Can you work these out from the model? Positions are in its coordinate system, mm. A direction names the side the tool comes from. Coordinates: 2 decimals unless noted, no trailing zeros. Write each loop counter-clockwise with the first axis right and the second up, starting at its lowest first coordinate (ties: lowest second). Pieces come first, ordered by that corner, then holes. Notation, with made-up numbers: (48, -32.5) -> (73, -32.5) arc R21 ccw to (73, -0.5) -> close; hole circle Ø8 at (50, 59). An arc over 180 degrees is marked (long way). Use one line per item in the form item = value.
```python
from build123d import *

# Parameters (mm, degrees)
SKETCH_1_W          = 52
SKETCH_1_H          = 17
SKETCH_1_W_2        = 17
SKETCH_1_H_2        = 52
EXTRUDE_1_DEPTH     = 15
SKETCH_8_W          = 11
SKETCH_8_H          = 54.414213562
SKETCH_8_W_2        = 54.414213562
SKETCH_8_H_2        = 11
CUT_EXTRUDE_2_DEPTH = 12
SKETCH_9_W          = 51.918987987
SKETCH_9_H          = 14
SKETCH_9_W_2        = 14
SKETCH_9_H_2        = 51.960636612
SKETCH_9_W_3        = 51.935924336
SKETCH_9_H_3        = 51.948438094
CUT_EXTRUDE_3_DEPTH = 10


with BuildPart() as part:
    # Эскиз1 → Бобышка-Вытянуть1 (new body)
    with BuildSketch(Plane.XY):
        with Locations((-46.52081528, 0)):
            Rectangle(SKETCH_1_W, SKETCH_1_H)
        Polygon((20.52081528, 8.5), (20.52081528, -8.5), (8.5, -20.52081528), (-8.5, -20.52081528), (-20.52081528, -8.5), (-20.52081528, 8.5), (-8.5, 20.52081528), (8.5, 20.52081528), align=None)
        with Locations((0, 46.52081528)):
            Rectangle(SKETCH_1_W_2, SKETCH_1_H_2)
        with Locations((46.52081528, 0)):
            Rectangle(SKETCH_1_W, SKETCH_1_H)
        with Locations((0, -46.52081528)):
            Rectangle(SKETCH_1_W_2, SKETCH_1_H_2)
    extrude(amount=EXTRUDE_1_DEPTH)

    # Эскиз8 → Вырез-Вытянуть2 (cut)
    with BuildSketch(Plane.XY.offset(15)):
        with Locations((0, 45.313708499)):
            Rectangle(SKETCH_8_W, SKETCH_8_H)
        Polygon((7.5, -18.106601718), (18.106601718, -7.5), (18.106601718, 7.5), (7.5, 18.106601718), (-7.5, 18.106601718), (-18.106601718, 7.5), (-18.106601718, -7.5), (-7.5, -18.106601718), align=None)
        with Locations((45.313708499, 0)):
            Rectangle(SKETCH_8_W_2, SKETCH_8_H_2)
        with Locations((0, -45.313708499)):
            Rectangle(SKETCH_8_W, SKETCH_8_H)
        with Locations((-45.313708499, 0)):
            Rectangle(SKETCH_8_W_2, SKETCH_8_H_2)
    extrude(amount=-CUT_EXTRUDE_2_DEPTH, mode=Mode.SUBTRACT)

    # Эскиз9 → Вырез-Вытянуть3 (cut)
    with BuildSketch(Plane.XY.offset(3)):
        with Locations((-46.561321287, 0)):
            Rectangle(SKETCH_9_W, SKETCH_9_H)
        with Locations((0, 46.540496974)):
            Rectangle(SKETCH_9_W_2, SKETCH_9_H_2)
        with Locations((46.552853112, 0)):
            Rectangle(SKETCH_9_W_3, SKETCH_9_H)
        with Locations((0, -46.546596233)):
            Rectangle(SKETCH_9_W_2, SKETCH_9_H_3)
    extrude(amount=CUT_EXTRUDE_3_DEPTH, mode=Mode.SUBTRACT)


solid = part.part
```
Q1. Thinking about a two-plate mould opening in Z: for faces 5 (the flat face through (72.521, 0, 2)), 6 (the flat face through (-7, 46, 8)), 7 (the flat face through (14, 14, 15)), which applies, released by +Z, released by -Z, zero draft, split by the parting line, or undercut?
Return value:
face_5 = zero draft
face_6 = undercut
face_7 = released by +Z
Q2. Will these pins go through, and if not, where does the flat tip stop? pin 1 (3.5 mm diameter, centred on x = 33, z = 6.5, fed in from -Y); pin 2 (3.5 mm diameter, centred on y = -50, z = 7.5, fed in from +X); pin 3 (12 mm diameter, centred on x = -10, y = -21, fed in from -Z); pin 4 (0.8 mm diameter, centred on x = 6.5, z = 7, fed in from -Y).
Return value:
pin_1 = -8.5
pin_2 = 8.5
pin_3 = 0
pin_4 = -20.57
Q3. For faces 1 (the flat face through (46, -7, 8)), 2 (the flat face through (5.5, -41, 14)), 3 (the flat face through (0, 0, 3)), 4 (the flat face through (-47, 8.5, 7)), which set-ups out of +Z, -Z, +X, -X, +Y, -Y let a thin tool reach every point of the face, with its end or its side?
Return value:
face_1 = +X
face_2 = +Z, +Y, -Y
face_3 = none
face_4 = +Z, -Z, -X, +Y
Q4. Suppose I cut it at D-D (y = 11.5). Write out the boundary of the cut face in (x, z), then the cut area to 3 significant figures.
Return value:
outline = (-17.52, 0) -> (17.52, 0) -> (17.52, 15) -> (14.11, 15) -> (14.11, 3) -> (-14.11, 3) -> (-14.11, 15) -> (-17.52, 15) -> close
area = 187 mm2
Q5. If I drill on line 1 (Y direction, x = -30.5, z = 12.5); line 2 (X direction, y = 36.5, z = 13.75), over which ranges is the centre line in solid material (lowest first)? Write a range as from..to.
Return value:
line_1 = -8.5..-7, 7..8.5
line_2 = -8.5..-5.5, 5.5..8.5
Q6. Suppose I cut it at C-C (z = 10.25). Give the number of separate pieces and of enclosed holes in the cut face, then the cut area to 4 significant figures.
Return value:
separate_pieces = 4
enclosed_holes = 0
area = 827.5 mm2
Q7. Suppose I cut it at A-A (y = -43.5). Write out the boundary of the cut face in (x, z), then the cut area to 3 significant figures.
Return value:
outline = (-8.5, 0) -> (8.5, 0) -> (8.5, 15) -> (5.5, 15) -> (5.5, 13) -> (7, 13) -> (7, 3) -> (-7, 3) -> (-7, 13) -> (-5.5, 13) -> (-5.5, 15) -> (-8.5, 15) -> close
area = 93.0 mm2
